Input: part model. Units: mm. Frame: model coordinates. A direction names the side the tool comes from. Coordinates: 2 decimals unless noted, no trailing zeros. Write each loop counter-clockwise with the first axis right and the second up, starting at its lowest first coordinate (ties: lowest second). Pieces come first, ordered by that corner, then holes.
1) Section query A-A (x = 0). Output: boundary loops of the cut face in (y, z).
2) Section query C-C (z = 11.25). Output: boundary loops of the cut face in (x, y), then the cut area to 3 significant figures.
3) Set-up query: faces 1 (the cylindrical face through (0, -1, 7)), 2 (the flat face through (0, 0, 16)). Return all of +Z, -Z, +X, -X, +Y, -Y with unobstructed straight access to the full face (end or side cutting, diameter ignored); none if empty.
4) Line query: L1, parallel to Z at x = -0.45, y = 1.2; L2, parallel to Y at x = 0.6, z = 10.25; L3, parallel to Y at x = 0.05, z = 6.5. Output: solid intervals per line, ascending.
5) Section query D-D (z = 14.75). Output: boundary loops of the cut face in (x, y), then the cut area to 3 significant figures.
6) Pin query (flat end, axial travel): pin 1 Ø1 at (y, z) = (-0.5, 7) entering from -X; pin 2 Ø1 at (x, y) = (1, 0) entering from -Z. Return the tip coordinate at first contact, or that it passes through.
from build123d import *

# Parameters (mm, degrees)
CROQUIS1_R              = 1
SALIENTE_EXTRUIR1_DEPTH = 14
CROQUIS2_R              = 1.5
SALIENTE_EXTRUIR2_DEPTH = 2
CHAFL_N1_SIZE           = 0.2


with BuildPart() as part:
    # Croquis1 → Saliente-Extruir1 (new body)
    with BuildSketch(Plane.XY):
        Circle(CROQUIS1_R)
    extrude(amount=SALIENTE_EXTRUIR1_DEPTH)

    # Croquis2 → Saliente-Extruir2 (add)
    with BuildSketch(Plane.XY.offset(14)):
        Circle(CROQUIS2_R)
    extrude(amount=SALIENTE_EXTRUIR2_DEPTH)

    # Chaflán1
    chafl_n1_edges = [part.edges().sort_by_distance(p)[0] for p in [
        (-1, 0, 0),
    ]]
    chamfer(chafl_n1_edges, length=CHAFL_N1_SIZE)


solid = part.part
Answer:
1. outline: (-1.5, 14) - (-1, 14) - (-1, 0.2) - (-0.8, 0) - (0.8, 0) - (1, 0.2) - (1, 14) - (1.5, 14) - (1.5, 16) - (-1.5, 16) - close
2. outline: circle Ø2 at (0, 0)
2. area: 3.14 mm2
3. face 1: -Z
3. face 2: +Z, +X, -X, +Y, -Y
4. L1: z = 14 to 16
4. L2: y = -0.8 to 0.8
4. L3: y = -1 to 1
5. outline: circle Ø3 at (0, 0)
5. area: 7.07 mm2
6. pin 1: stops at x = -1
6. pin 2: stops at z = 0
